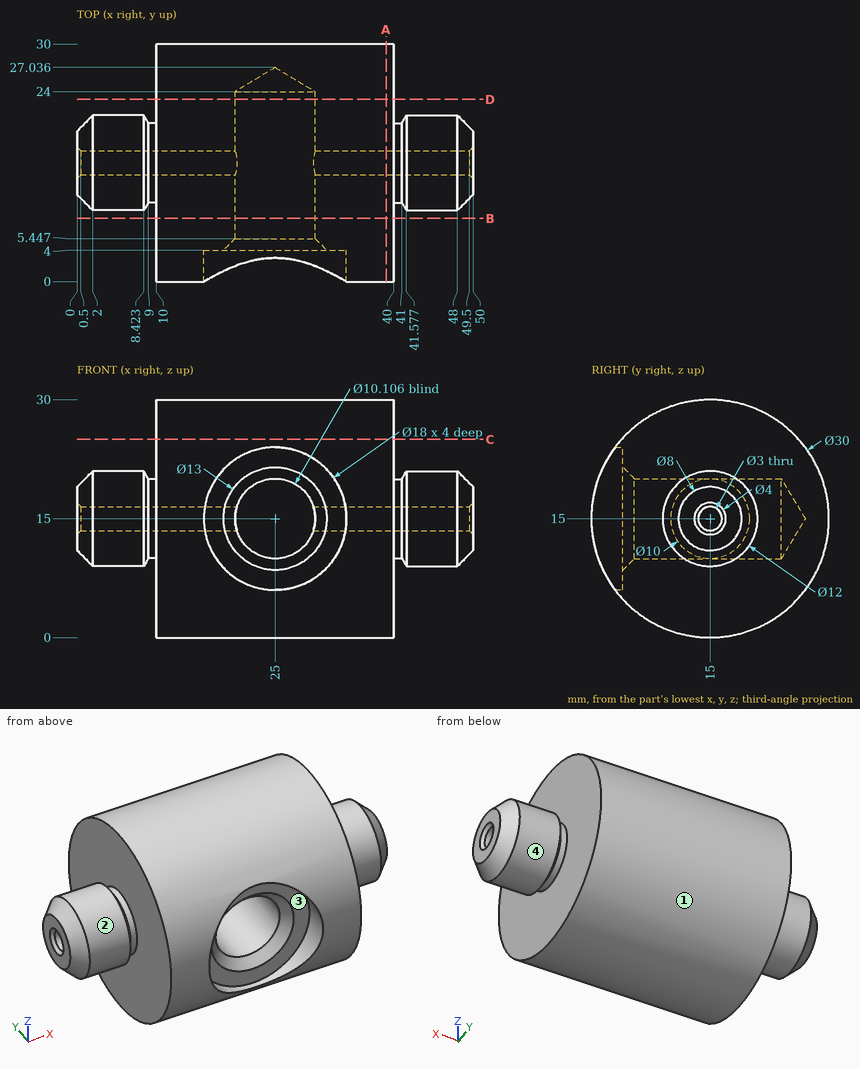
The drawing under review shows one solid part. Ordinate dimensions are in mm from its lowest x, y, z. A direction names the side the tool comes from. Coordinates: 2 decimals unless noted, no trailing zeros. Loops run counter-clockwise (first coordinate to the right, second up) from the corner with the lowest first, then second, coordinate; pieces in that order, holes last. Notation, with made-up numbers: (-11, -39.75) -> (17, -39.75) arc R33 cw to (17, -3.75) -> close; hole circle Ø10 at (34, -19.5). An arc over 180 degrees is marked (long way). Answer as a JSON object with one key per item and string values.
Q1. Take a section at D-D on y = 23. Give the boundary of the cut face in (x, z).
Answer block:
{"outline": "(10, 2.31) -> (40, 2.31) -> (40, 27.69) -> (10, 27.69) -> close; hole circle Ø10.11 at (25, 15)"}
Q2. Take a section at C-C on z = 25. Give the boundary of the cut face in (x, y).
Answer block:
{"outline": "(10, 3.82) -> (40, 3.82) -> (40, 26.18) -> (10, 26.18) -> close"}
Q3. Take a section at A-A on x = 39. Give the boundary of the cut face in (y, z), plus the area to 3 significant figures.
Answer block:
{"outline": "circle Ø30 at (15, 15); hole circle Ø3 at (15, 15)", "area": "700 mm^2"}
Q4. Tool access review of the marked faces 1, 2, 3 and 4: name each direction out of +Z, -Z, +X, -X, +Y, -Y from which nothing blocks a thin tool from reaching the whole face with its end or side.
Answer block:
{"face 1": "+X, -X", "face 2": "-X", "face 3": "-Y", "face 4": "+X"}
Q5. To check wall thickness, follow L1, parallel to Z at x = 39, y = 15; L2, parallel to Z at x = 8, y = 15; L3, parallel to X at y = 26.5, z = 18. State the ranges of each line that lie inside material, in increasing order.
Answer block:
{"L1": "z = 0 to 13.5, 16.5 to 30", "L2": "z = 9 to 13.5, 16.5 to 21", "L3": "x = 10 to 40"}
Q6. Clearance check with flat-ended pins moving along their axes: pin 1 Ø1.5 at (x, z) = (19.5, 27) entering from +Y; pin 2 Ø10 at (x, y) = (36, 3) entering from -Z; pin 3 Ø12 at (x, y) = (20, 4.5) entering from -Z; pin 4 Ø8 at (x, z) = (42.5, 14.5) entering from +Y. State where each tip first meets the part, or that it passes through.
Answer block:
{"pin 1": "stops at y = 24.92", "pin 2": "stops at z = 1.73", "pin 3": "stops at z = 0.69", "pin 4": "stops at y = 30"}
Q7. Take a section at B-B on y = 8. Give the boundary of the cut face in (x, z).
Answer block:
{"outline": "(10, 1.73) -> (40, 1.73) -> (40, 28.27) -> (10, 28.27) -> close; hole circle Ø10.11 at (25, 15)"}
